```python
from build123d import *

# Parameters (mm, degrees)
F0_R     = 2.5
F1_DEPTH = 25


with BuildPart() as f1:
    # F0 (on Right) → F1 (new body)
    with BuildSketch(Plane.YZ):
        with BuildLine():
            Line((4.5, 4.5), (0, 4.5))
            ThreePointArc((0, 4.5), (-4.5, 0), (0, -4.5))
            Line((0, -4.5), (4.5, -4.5))
            Line((4.5, -4.5), (4.5, 4.5))
        make_face()
        Circle(F0_R, mode=Mode.SUBTRACT)
    extrude(amount=F1_DEPTH)


solid = f1.part
```
Check sheet for the modelled part. Datum: model origin and axes. Units: mm. Coordinates: 2 decimals unless noted, no trailing zeros. Write each loop counter-clockwise with the first axis right and the second up, starting at its lowest first coordinate (ties: lowest second). Pieces come first, ordered by that corner, then holes. Notation, with made-up numbers: M -24,-12 L 6,-12 A21 ccw 6,16 Z; hole C -27,31 d1. An arc over 180 degrees is marked long. Use one line per item in the form item = value.
Item 1: Gauge pin test, flat end, axial feed: pin 1 Ø1 at (x, y) = (7.5, -3) entering from +Z. Record the tip position at first contact, or that the pin passes through.
Answer below:
pin_1 = 3.74
Item 2: Sectioned sample at D-D, the plane z = 2.75. Record the cut outline in (x, y).
Answer below:
outline = M 0,-3.56 L 25,-3.56 L 25,4.5 L 0,4.5 Z
Item 3: Sectioned sample at B-B, the plane y = -1.5. Record the cut outline in (x, z).
Answer below:
outline = M 0,-4.24 L 25,-4.24 L 25,-2 L 0,-2 Z; M 0,2 L 25,2 L 25,4.24 L 0,4.24 Z
Item 4: Sectioned sample at C-C, the plane x = 21.5. Record the cut outline in (y, z).
Answer below:
outline = M 0,-4.5 L 4.5,-4.5 L 4.5,4.5 L 0,4.5 A4.5 ccw Z; hole C 0,0 d5
Item 5: Sectioned sample at A-A, the plane z = 0. Record the cut outline in (x, y).
Answer below:
outline = M 0,-4.5 L 25,-4.5 L 25,-2.5 L 0,-2.5 Z; M 0,2.5 L 25,2.5 L 25,4.5 L 0,4.5 Z
Item 6: Material ranges on L1, parallel to Z at x = 16.25, y = 2; L2, parallel to Z at x = 14.75, y = 1.5; L3, parallel to Y at x = 18.5, z = -0.5, recorded low to high. Write a range as from..to.
Answer below:
L1 = -4.5..-1.5, 1.5..4.5
L2 = -4.5..-2, 2..4.5
L3 = -4.47..-2.45, 2.45..4.5
Item 7: Release check for a two-part mould opening along Y. For faces 1 (the face through (25, 2, -2)), 2 (the face through (12, 4.5, 0)), 3 (the face through (12.32, -0.54, -2.44)) record: pulls with the +Y half, pulls with the -Y half, needs draft (parallel to the pull), parting line crosses it, or undercut.
Answer below:
face_1 = needs draft
face_2 = pulls with the +Y half
face_3 = undercut
